from build123d import *

# Parameters (mm, degrees)
CROQUIS1_R              = 55
CROQUIS1_W              = 45
CROQUIS1_H              = 15
SALIENTE_EXTRUIR1_DEPTH = 10
CROQUIS2_W              = 10
CROQUIS2_H              = 30
SALIENTE_EXTRUIR2_DEPTH = 95
CROQUIS3_R              = 1.5
CORTAR_EXTRUIR1_DEPTH   = 50
CORTAR_EXTRUIR2_DEPTH   = 10
CROQUIS5_R              = 2.5
CORTAR_EXTRUIR3_DEPTH   = 85
CROQUIS7_R              = 2.5
SALIENTE_EXTRUIR3_DEPTH = 5
CORTAR_EXTRUIR4_DEPTH   = 10
CROQUIS10_R             = 2.575
CROQUIS11_OUTSIDE_W     = 149.536
CROQUIS11_OUTSIDE_H     = 144.536
CROQUIS11_OUTSIDE_W_2   = 10
CROQUIS11_OUTSIDE_H_2   = 100
CORTAR_EXTRUIR5_DEPTH   = 105.5
CROQUIS12_OUTSIDE_W     = 40.072
CROQUIS12_OUTSIDE_H     = 128.052
CROQUIS12_OUTSIDE_W_2   = 10
CROQUIS12_OUTSIDE_H_2   = 30
CORTAR_EXTRUIR6_DEPTH   = 10
SALIENTE_EXTRUIR4_DEPTH = 50
CORTAR_EXTRUIR7_DEPTH   = 30
CROQUIS18_OUTSIDE_W     = 40.218
CROQUIS18_OUTSIDE_H     = 70.744
CROQUIS18_OUTSIDE_W_2   = 10
CROQUIS18_OUTSIDE_H_2   = 30
CORTAR_EXTRUIR8_DEPTH   = 5


with BuildPart() as part:
    # Croquis1 → Saliente-Extruir1 (new body)
    with BuildSketch(Plane.XY):
        Circle(CROQUIS1_R)
        with Locations((0, -2.5)):
            Rectangle(CROQUIS1_W, CROQUIS1_H, mode=Mode.SUBTRACT)
    extrude(amount=SALIENTE_EXTRUIR1_DEPTH)

    # Croquis2 → Saliente-Extruir2 (add)
    with BuildSketch(Plane.XY.offset(10)):
        with Locations((30, 0)):
            Rectangle(CROQUIS2_W, CROQUIS2_H)
    extrude(amount=SALIENTE_EXTRUIR2_DEPTH)

    # Croquis3 → Cortar-Extruir1 (cut)
    with BuildSketch(Plane.XZ.offset(15)):
        with Locations((30, 100)):
            Circle(CROQUIS3_R)
    extrude(amount=-CORTAR_EXTRUIR1_DEPTH, mode=Mode.SUBTRACT)

    # Croquis4 → Cortar-Extruir2 (cut)
    with BuildSketch(Plane.XZ.offset(15)):
        Polygon((35, 85), (25, 55), (25, 95), (25, 105), (35, 105), align=None)
    cortar_extruir2 = extrude(amount=-CORTAR_EXTRUIR2_DEPTH, mode=Mode.SUBTRACT)

    # Simetría1: Cortar-Extruir2 across plane
    add(cortar_extruir2.mirror(Plane.ZX), mode=Mode.SUBTRACT)

    # Croquis5 → Cortar-Extruir3 (cut, symmetric)
    with BuildSketch(Plane.XZ.offset(-5)):
        with Locations(Location((0, 5, 0), (0, 0, 270))):
            Circle(CROQUIS5_R)
    extrude(amount=CORTAR_EXTRUIR3_DEPTH, both=True, mode=Mode.SUBTRACT)

    # Croquis7 → Saliente-Extruir3 (add)
    with BuildSketch(Plane.XY.offset(10)):
        with Locations((0, 48.5)):
            Circle(CROQUIS7_R)
    extrude(amount=SALIENTE_EXTRUIR3_DEPTH)

    # Croquis8 → Cortar-Extruir4 (cut)
    with BuildSketch(Plane.XY.offset(10)):
        with BuildLine():
            Line((8.999999995, 39.891287847), (8.999999995, 38.6))
            Line((8.999999995, 38.6), (7.708712148, 38.6))
            ThreePointArc((7.708712148, 38.6), (7.499999995, 37.6), (7.708712148, 36.6))
            Line((7.708712148, 36.6), (8.999999995, 36.6))
            Line((8.999999995, 36.6), (8.999999995, 35.308712153))
            ThreePointArc((8.999999995, 35.308712153), (9.999999995, 35.1), (10.999999995, 35.308712153))
            Line((10.999999995, 35.308712153), (10.999999995, 36.6))
            Line((10.999999995, 36.6), (12.291287843, 36.6))
            ThreePointArc((12.291287843, 36.6), (12.499999995, 37.6), (12.291287843, 38.6))
            Line((12.291287843, 38.6), (10.999999995, 38.6))
            Line((10.999999995, 38.6), (10.999999995, 39.891287847))
            ThreePointArc((10.999999995, 39.891287847), (9.999999995, 40.1), (8.999999995, 39.891287847))
        make_face()
        with BuildLine():
            Line((-7.708712157, 36.6), (-9.000000005, 36.6))
            Line((-9.000000005, 36.6), (-9.000000005, 35.308712153))
            ThreePointArc((-9.000000005, 35.308712153), (-10.000000005, 35.1), (-11.000000005, 35.308712153))
            Line((-11.000000005, 35.308712153), (-11.000000005, 36.6))
            Line((-11.000000005, 36.6), (-12.291287852, 36.6))
            ThreePointArc((-12.291287852, 36.6), (-12.500000005, 37.6), (-12.291287852, 38.6))
            Line((-12.291287852, 38.6), (-11.000000005, 38.6))
            Line((-11.000000005, 38.6), (-11.000000005, 39.891287847))
            ThreePointArc((-11.000000005, 39.891287847), (-10.000000005, 40.1), (-9.000000005, 39.891287847))
            Line((-9.000000005, 39.891287847), (-9.000000005, 38.6))
            Line((-9.000000005, 38.6), (-7.708712157, 38.6))
            ThreePointArc((-7.708712157, 38.6), (-7.500000005, 37.6), (-7.708712157, 36.6))
        make_face()
        with BuildLine():
            Line((-7.708712153, -35.749999986), (-9, -35.749999986))
            Line((-9, -35.749999986), (-9, -37.041287833))
            ThreePointArc((-9, -37.041287833), (-10, -37.249999986), (-11, -37.041287833))
            Line((-11, -37.041287833), (-11, -35.749999986))
            Line((-11, -35.749999986), (-12.291287847, -35.749999986))
            ThreePointArc((-12.291287847, -35.749999986), (-12.5, -34.749999986), (-12.291287847, -33.749999986))
            Line((-12.291287847, -33.749999986), (-11, -33.749999986))
            Line((-11, -33.749999986), (-11, -32.458712138))
            ThreePointArc((-11, -32.458712138), (-10, -32.249999986), (-9, -32.458712138))
            Line((-9, -32.458712138), (-9, -33.749999986))
            Line((-9, -33.749999986), (-7.708712153, -33.749999986))
            ThreePointArc((-7.708712153, -33.749999986), (-7.5, -34.749999986), (-7.708712153, -35.749999986))
        make_face()
        with BuildLine():
            Line((8.999999991, -35.749999986), (8.999999991, -37.041287833))
            ThreePointArc((8.999999991, -37.041287833), (9.999999991, -37.249999986), (10.999999991, -37.041287833))
            Line((10.999999991, -37.041287833), (10.999999991, -35.749999986))
            Line((10.999999991, -35.749999986), (12.291287838, -35.749999986))
            ThreePointArc((12.291287838, -35.749999986), (12.499999991, -34.749999986), (12.291287838, -33.749999986))
            Line((12.291287838, -33.749999986), (10.999999991, -33.749999986))
            Line((10.999999991, -33.749999986), (10.999999991, -32.458712138))
            ThreePointArc((10.999999991, -32.458712138), (9.999999991, -32.249999986), (8.999999991, -32.458712138))
            Line((8.999999991, -32.458712138), (8.999999991, -33.749999986))
            Line((8.999999991, -33.749999986), (7.708712143, -33.749999986))
            ThreePointArc((7.708712143, -33.749999986), (7.499999991, -34.749999986), (7.708712143, -35.749999986))
            Line((7.708712143, -35.749999986), (8.999999991, -35.749999986))
        make_face()
    extrude(amount=-CORTAR_EXTRUIR4_DEPTH, mode=Mode.SUBTRACT)

    # Croquis10 → Cortar-Revolución1 (revolve, cut)
    with BuildSketch(Plane(origin=(0, 0, 0), x_dir=(1, 0, 0), z_dir=(0, 1, 0))):
        with Locations((-55, -5)):
            Circle(CROQUIS10_R)
    revolve(axis=Axis((0, 0, 0), (0, 0, 1)), mode=Mode.SUBTRACT)

    # Croquis11 outside → Cortar-Extruir5 (cut, symmetric)
    with BuildSketch(Plane(origin=(0, 15, 0), x_dir=(1, 0, 0), z_dir=(0, 1, 0))):
        with Locations((0, -52.5)):
            Rectangle(CROQUIS11_OUTSIDE_W, CROQUIS11_OUTSIDE_H)
        with Locations((30, -55)):
            Rectangle(CROQUIS11_OUTSIDE_W_2, CROQUIS11_OUTSIDE_H_2, mode=Mode.SUBTRACT)
    extrude(amount=CORTAR_EXTRUIR5_DEPTH, both=True, mode=Mode.SUBTRACT)

    # Croquis12 outside → Cortar-Extruir6 (cut)
    with BuildSketch(Plane.XY.offset(10)):
        with Locations((30, 0)):
            Rectangle(CROQUIS12_OUTSIDE_W, CROQUIS12_OUTSIDE_H)
        with Locations((30, 0)):
            Rectangle(CROQUIS12_OUTSIDE_W_2, CROQUIS12_OUTSIDE_H_2, mode=Mode.SUBTRACT)
    extrude(amount=-CORTAR_EXTRUIR6_DEPTH, mode=Mode.SUBTRACT)

    # Croquis15 → Saliente-Extruir4 (add)
    with BuildSketch(Plane(origin=(0, 0, 5), x_dir=(-1, 0, 0), z_dir=(0, 0, -1))):
        Polygon((-30, 15), (-20.877471703, 23.230682918), (-19.064126659, 21.220850729), (-25, 9.458219088), align=None)
    saliente_extruir4 = extrude(amount=-SALIENTE_EXTRUIR4_DEPTH)

    # Croquis17 → Cortar-Extruir7 (cut)
    with BuildSketch(Plane(origin=(23.729923141, 11.975025866, 0), x_dir=(0, 0, 1), z_dir=(-0.8927647254437483, -0.4505231903058363, 0))):
        Polygon((55, 2.599765556), (10, 10.356395812), (-8.093174243, 24.440719527), (32.70757592, 13.533993104), (58.299435985, 13.533993104), align=None)
    cortar_extruir7 = extrude(amount=-CORTAR_EXTRUIR7_DEPTH, mode=Mode.SUBTRACT)

    # Simetría2: Saliente-Extruir4, Cortar-Extruir7 across plane
    add(saliente_extruir4.mirror(Plane.ZX))
    add(cortar_extruir7.mirror(Plane.ZX), mode=Mode.SUBTRACT)

    # Croquis18 outside → Cortar-Extruir8 (cut)
    with BuildSketch(Plane(origin=(0, 0, 5), x_dir=(-1, 0, 0), z_dir=(0, 0, -1))):
        with Locations((-27.032, 0)):
            Rectangle(CROQUIS18_OUTSIDE_W, CROQUIS18_OUTSIDE_H)
        with Locations((-30, 0)):
            Rectangle(CROQUIS18_OUTSIDE_W_2, CROQUIS18_OUTSIDE_H_2, mode=Mode.SUBTRACT)
    extrude(amount=-CORTAR_EXTRUIR8_DEPTH, mode=Mode.SUBTRACT)


solid = part.part
Read the model definition and answer for the solid it produces. Units are mm, in the model's axes. A direction names the side the tool comes from. Coordinates: 2 decimals unless noted, no trailing zeros. Loops run counter-clockwise (first coordinate to the right, second up) from the corner with the lowest first, then second, coordinate; pieces in that order, holes last. Notation, with made-up numbers: (4, -39.5) -> (45, -39.5) arc R12 ccw to (45, -24.5) -> close; hole circle Ø7 at (61.25, 0). An arc over 180 degrees is marked (long way). Answer in a Markdown table with one row per item.
Item 1: A cutting plane is placed at C-C on x = 26.25. Determine the outline of the cut face in (y, z).
Returned:
| item | result |
|---|---|
| outline | (-18.38, 10) -> (-15, 10) -> (-15, 5) -> (15, 5) -> (15, 10) -> (18.38, 10) -> (18.38, 43.48) -> (16.16, 55) -> (15, 55) -> (15, 58.75) -> (5, 58.75) -> (5, 105) -> (-5, 105) -> (-5, 58.75) -> (-15, 58.75) -> (-15, 55) -> (-16.16, 55) -> (-18.38, 43.48) -> close |
Item 2: Straight lines are drawn through the part: line 1 along X through (y, z) = (-1, 100); line 2 along Z through (x, y) = (30, 1.75); line 3 along Y through (x, z) = (25.5, 82). For each, find the intervals that lie inside material, in ascending order. Write a range as [from, to].
Returned:
| item | result |
|---|---|
| line 1 | x = [25, 28.5], [31.5, 35] |
| line 2 | z = [5, 98.5], [101.5, 105] |
| line 3 | y = [-5, 5] |
Item 3: Each of these flat-tipped pins is pushed along its axis until it touches: P1, Ø4, axis at x = 27.5, z = 71, coming from the -Y side; P2, Ø5, axis at x = 28.5, z = 77.5, coming from the +Y side; P3, Ø8, axis at x = 30.5, z = 76.5, coming from the -Y side. Where does it stop, or does it pass through?
Returned:
| item | result |
|---|---|
| P1 | stops at y = -5 |
| P2 | stops at y = 5 |
| P3 | stops at y = -15 |
Item 4: For a pull along Z with two mould halves and no side action, classify faces 6 (the flat face through (30, 0, 105)), 7 (the flat face through (26.81, 17.88, 27.18)), 8 (the cylindrical face through (29.805, -0.07, 101.487)) as released by +Z, released by -Z, zero draft, split by the parting line, or undercut.
Returned:
| item | result |
|---|---|
| face 6 | released by +Z |
| face 7 | zero draft |
| face 8 | undercut |
Item 5: For faces 1 (the flat face through (24.6, -14.1, 55)), 2 (the flat face through (24.6, 14.1, 55)), 3 (the flat face through (26.81, -17.88, 27.18)), 4 (the flat face through (22.65, -14.115, 27.185)), 5 (the flat face through (35, 0, 45)), determine the directions among +Z, -Z, +X, -X, +Y, -Y from which every point of the face is accessible in a straight line to the end or side of a thin tool.
Returned:
| item | result |
|---|---|
| face 1 | +Z, -X, -Y |
| face 2 | +Z, -X, +Y |
| face 3 | +Z, -Z, +X, -Y |
| face 4 | +Z, -Z, -X |
| face 5 | +Z, -Z, +X, +Y, -Y |
Item 6: A cutting plane is placed at A-A on z = 100. Determine the outline of the cut face in (x, y).
Returned:
| item | result |
|---|---|
| outline | (25, -5) -> (28.5, -5) -> (28.5, 5) -> (25, 5) -> close; (31.5, -5) -> (35, -5) -> (35, 5) -> (31.5, 5) -> close |
Item 7: A cutting plane is placed at B-B on y = -3. Determine the outline of the cut face in (x, z), plus the area to 3 significant figures.
Returned:
| item | result |
|---|---|
| outline | (25, 5) -> (35, 5) -> (35, 105) -> (25, 105) -> close; hole circle Ø3 at (30, 100) |
| area | 993 mm^2 |
Item 8: A cutting plane is placed at D-D on z = 34. Determine the outline of the cut face in (x, y), plus the area to 3 significant figures.
Returned:
| item | result |
|---|---|
| outline | (20.93, -17.53) -> (24.95, -19.56) -> (30, -15) -> (35, -15) -> (35, 15) -> (30, 15) -> (24.95, 19.56) -> (20.93, 17.53) -> (25, 9.46) -> (25, -9.46) -> close |
| area | 364 mm^2 |
